```python
from build123d import *

# Parameters (mm, degrees)
F0_R     = 22.5
F1_DEPTH = 2
F2_DEPTH = 8


with BuildPart() as f1:
    # F0 (on Top) → F1 (new body)
    with BuildSketch(Plane.XY):
        Circle(F0_R)
        with BuildLine():
            Line((5, 3.297524), (5, -4.202476))
            ThreePointArc((5, -4.202476), (0, -9.202476), (-5, -4.202476))
            Line((-5, -4.202476), (-5, 3.297524))
            ThreePointArc((-5, 3.297524), (0, 8.297524), (5, 3.297524))
        make_face(mode=Mode.SUBTRACT)
        with BuildLine():
            ThreePointArc((-5, -4.202476), (-4.557189, -2.145287), (-3.307189, -0.452476))
            ThreePointArc((-3.307189, -0.452476), (-4.557189, 1.240335), (-5, 3.297524))
            Line((-5, 3.297524), (-5, -4.202476))
        make_face()
        with BuildLine():
            ThreePointArc((-2.5, 3.297524), (0, 5.797524), (2.5, 3.297524))
            Line((2.5, 3.297524), (2.5, 0.127651))
            ThreePointArc((2.5, 0.127651), (2.918047, -0.142303), (3.307189, -0.452476))
            ThreePointArc((3.307189, -0.452476), (4.557189, 1.240335), (5, 3.297524))
            ThreePointArc((5, 3.297524), (0, 8.297524), (-5, 3.297524))
            ThreePointArc((-5, 3.297524), (-4.557189, 1.240335), (-3.307189, -0.452476))
            ThreePointArc((-3.307189, -0.452476), (-2.918047, -0.142303), (-2.5, 0.127651))
            Line((-2.5, 0.127651), (-2.5, 3.297524))
        make_face()
        with BuildLine():
            ThreePointArc((5, 3.297524), (4.557189, 1.240335), (3.307189, -0.452476))
            ThreePointArc((3.307189, -0.452476), (4.557189, -2.145287), (5, -4.202476))
            Line((5, -4.202476), (5, 3.297524))
        make_face()
    extrude(amount=F1_DEPTH)

    # F0 (on Top) → F2 (join)
    with BuildSketch(Plane.XY):
        Circle(F0_R)
        with BuildLine():
            Line((5, 3.297524), (5, -4.202476))
            ThreePointArc((5, -4.202476), (0, -9.202476), (-5, -4.202476))
            Line((-5, -4.202476), (-5, 3.297524))
            ThreePointArc((-5, 3.297524), (0, 8.297524), (5, 3.297524))
        make_face(mode=Mode.SUBTRACT)
    extrude(amount=F2_DEPTH)


solid = f1.part
```
Input: part model. Units: mm. Frame: model coordinates. A direction names the side the tool comes from. Coordinates: 2 decimals unless noted, no trailing zeros. Write each loop counter-clockwise with the first axis right and the second up, starting at its lowest first coordinate (ties: lowest second). Pieces come first, ordered by that corner, then holes. Notation, with made-up numbers: M 58,19.5 L 73,19.5 A13 cw 73,36.5 Z; hole C -15.5,13.25 d6. An arc over 180 degrees is marked long. Use one line per item in the form item = value.
Q1. Section D-D (z = 1). Return loops of the section in (x, y).
Answer below:
outline = C 0,0 d45; hole M -5,-4.2 A5 ccw 5,-4.2 A5 ccw 3.31,-0.45 A5 ccw 2.5,0.13 L 2.5,3.3 A2.5 ccw -2.5,3.3 L -2.5,0.13 A5 ccw -3.31,-0.45 A5 ccw Z
Q2. Draft query along Y for faces 1 (the face through (10.382, -19.961, 3.944)), 2 (the face through (-5.3, 0.3, 8)), 3 (the face through (2.5, 2, 1)). Return one class per face: released by +Y, released by -Y, zero draft, split by the parting line, or undercut.
Answer below:
face_1 = split by the parting line
face_2 = zero draft
face_3 = undercut
Q3. Section A-A (x = 0). Return loops of the section in (y, z), plus the area to 3 significant figures.
Answer below:
outline = M -22.5,0 L -9.2,0 L -9.2,8 L -22.5,8 Z; M 5.8,0 L 22.5,0 L 22.5,8 L 8.3,8 L 8.3,2 L 5.8,2 Z
area = 225 mm²
Q4. Set-up query: faces 4 (the face through (5, 0, 0)), 5 (the face through (-0.055, 5.797, 0.986)), 6 (the face through (-0.11, 8.296, 4.958)). Return all of +Z, -Z, +X, -X, +Y, -Y with unobstructed straight access to the full face (end or side cutting, diameter ignored); none if empty.
Answer below:
face_4 = -Z, +X, -X, +Y, -Y
face_5 = +Z, -Z
face_6 = +Z
Q5. Section C-C (y = -3.5). Return loops of the section in (x, z), plus the area to 3 significant figures.
Answer below:
outline = M -22.23,0 L -4.95,0 L -4.95,2 L -5,2 L -5,8 L -22.23,8 Z; M 4.95,0 L 22.23,0 L 22.23,8 L 5,8 L 5,2 L 4.95,2 Z
area = 276 mm²
Q6. Material intervals for probe 1 along Z at (x, y) = (2.5, 4); probe 2 along Y at (x, z) = (-4.5, 4.25); probe 3 along X at (y, z) = (1, 6), sorted ascending. Write a range as from..to.
Answer below:
probe_1 = 0..2
probe_2 = -22.05..-6.38, 5.48..22.05
probe_3 = -22.48..-5, 5..22.48
Q7. Section B-B (z = 7). Return loops of the section in (x, y).
Answer below:
outline = C 0,0 d45; hole M -5,-4.2 A5 ccw 5,-4.2 L 5,3.3 A5 ccw -5,3.3 Z
Q8. First-contact query: pin 1 (3 mm diameter, centred on x = 11.5, z = 3, fed in from +Y); pin 2 (4 mm diameter, centred on y = 9, z = 5.5, fed in from -X); pin 3 (2 mm diameter, centred on x = -15.5, z = 7, fed in from -Y). Flat tips, straight axial feed; report the tip coordinate or a pass-through.
Answer below:
pin_1 = 20.16
pin_2 = -21.38
pin_3 = -17.2
